Check sheet for the drawn part. Datum: minimum x, y, z corner. Units: mm. Give positions to 0.01 mm unless a question says otherwise; leave off trailing zeros. Write each loop counter-clockwise with the first axis right and the second up, starting at its lowest first coordinate (ties: lowest second). Pieces come first, ordered by that corner, then holes.
(1) Cross-section at A-A (y = 50). Record the boundary of the cut face in (x, z).
(2) Cross-section at B-B (x = 325). Record the boundary of the cut face in (y, z).
(3) Cross-section at C-C (z = 12.5). Record the boundary of the cut face in (x, y).
(4) Thickness scan on line 1 along X through (y, z) = (50, 50); line 2 along Y through (x, z) = (25, 36); line 3 along Y through (x, z) = (25, 51.5). Record the ranges inside material, lowest first.
(5) Depth check by flat-ended pin: P1, Ø2, axis at x = 188.5, z = 49, coming from the -Y side. Enter the tip coordinate at first touch or a pass-through.
(6) Cross-section at D-D (x = 275). Record the boundary of the cut face in (y, z), and give its area (3 significant figures).
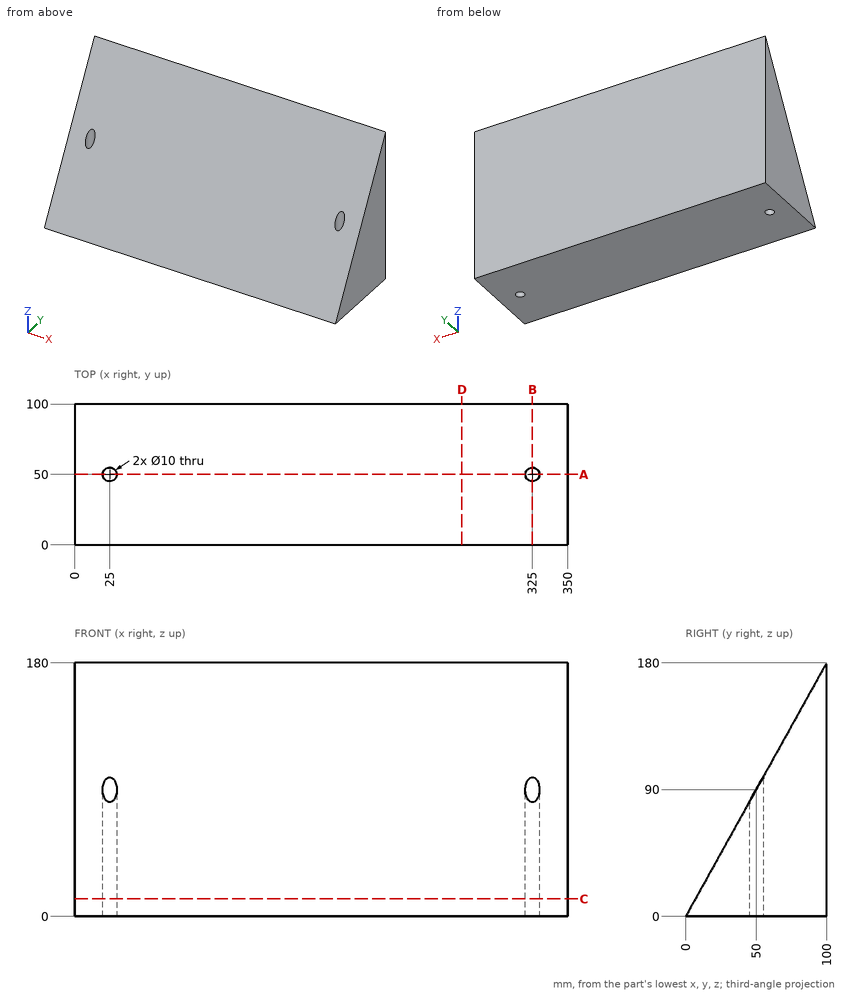
Reply:
1. outline: (0, 0) - (20, 0) - (20, 90) - (0, 90) - close; (30, 0) - (320, 0) - (320, 90) - (30, 90) - close; (330, 0) - (350, 0) - (350, 90) - (330, 90) - close
2. outline: (0, 0) - (45, 0) - (45, 81) - close; (55, 0) - (100, 0) - (100, 180) - (55, 99) - close
3. outline: (0, 6.94) - (350, 6.94) - (350, 100) - (0, 100) - close; hole circle Ø10 at (25, 50); hole circle Ø10 at (325, 50)
4. line 1: x = 0 to 20, 30 to 320, 330 to 350
4. line 2: y = 20 to 45, 55 to 100
4. line 3: y = 28.61 to 45, 55 to 100
5. P1: stops at y = 26.67
6. outline: (0, 0) - (100, 0) - (100, 180) - close
6. area: 9,000 mm2
